from build123d import *

# Parameters (mm, degrees)
F0_W     = 34.925
F0_H     = 1.5875
F1_DEPTH = 7.9375
F2_R     = 1.4097
F3_DEPTH = 1.5875


with BuildPart() as f1:
    # F0 (on Front) → F1 (new body)
    with BuildSketch(Plane.XZ):
        with Locations((27.560851, 10.8921)):
            Rectangle(F0_W, F0_H)
    extrude(amount=F1_DEPTH)

    # F2 (on face) → F3 (cut)
    with BuildSketch(Plane.XY.offset(11.68585)):
        with Locations((14.067101, -3.96875)):
            Circle(F2_R)
        with Locations((41.054601, -3.96875)):
            Circle(F2_R)
    extrude(amount=-F3_DEPTH, mode=Mode.SUBTRACT)


solid = f1.part
Geometry: final body of the model. Coordinates: model frame, mm. Round coordinates to 2 decimals unless told otherwise and drop trailing zeros. Loops run counter-clockwise (first coordinate to the right, second up) from the corner with the lowest first, then second, coordinate; pieces in that order, holes last. Notation, with made-up numbers: (6.25, 30.5) - (42.25, 30.5) arc R13 ccw to (42.25, 43.5) - close; hole circle Ø9 at (0.5, 16.25). An arc over 180 degrees is marked (long way). Write each question's results on one line, items separated by ' | '. Start each with the question number.
1) Line query: probe 1 along X at (y, z) = (-3, 10.3); probe 2 along X at (y, z) = (-5.25, 11.35); probe 3 along Y at (x, z) = (13, 10.6). Output: solid intervals per line, ascending. Write a range as [from, to].
2) Mould query, pull axis X, two halves, no side actions, for faces 1 (the face through (15.412, -3.545, 10.903)), 2 (the face through (45.023, -4, 11)), 3 (the face through (27, -4, 11.686)), 4 (the face through (10.098, -4, 11)). Classes: released by +X, released by -X, zero draft, split by the parting line, or undercut.
3) Cut plane C-C on z = 11. Return loops of the section in (x, y), then the cut area to 3 significant figures.
4) Cut plane B-B on y = -4.5. Return loops of the section in (x, z), then the cut area to 3 significant figures.
5) Cut plane A-A on x = 13.5. Return loops of the section in (y, z).
Verdict:
1) probe 1: x = [10.1, 13.04], [15.09, 40.03], [42.08, 45.02] | probe 2: x = [10.1, 13.48], [14.66, 40.47], [41.64, 45.02] | probe 3: y = [-7.94, -4.89], [-3.05, 0]
2) face 1: undercut | face 2: released by +X | face 3: zero draft | face 4: released by -X
3) outline: (10.1, -7.94) - (45.02, -7.94) - (45.02, 0) - (10.1, 0) - close; hole circle Ø2.82 at (14.07, -3.97); hole circle Ø2.82 at (41.05, -3.97) | area: 265 mm2
4) outline: (10.1, 10.1) - (12.76, 10.1) - (12.76, 11.69) - (10.1, 11.69) - close; (15.37, 10.1) - (39.75, 10.1) - (39.75, 11.69) - (15.37, 11.69) - close; (42.36, 10.1) - (45.02, 10.1) - (45.02, 11.69) - (42.36, 11.69) - close | area: 47.2 mm2
5) outline: (-7.94, 10.1) - (-5.26, 10.1) - (-5.26, 11.69) - (-7.94, 11.69) - close; (-2.68, 10.1) - (0, 10.1) - (0, 11.69) - (-2.68, 11.69) - close
